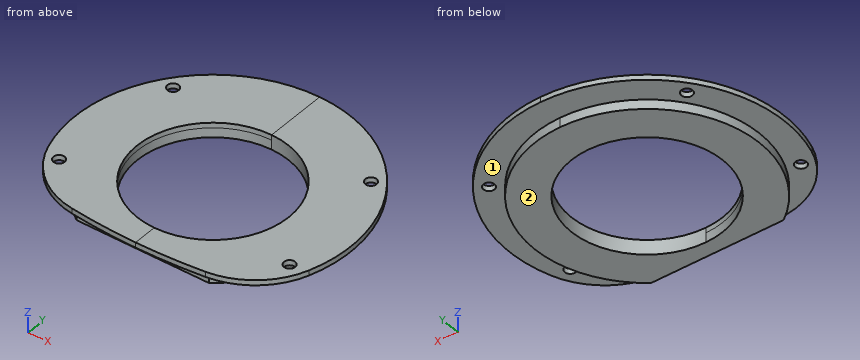
```python
from build123d import *

# Parameters (mm, degrees)
PAD_DEPTH    = 3
PAD001_DEPTH = 5.5
SKETCH002_R  = 3.25
POCKET_DEPTH = 5


with BuildPart() as part:
    # Sketch → Pad (new body)
    with BuildSketch(Plane.XY):
        with BuildLine():
            ThreePointArc((0, -44), (44, 0), (0, 44))
            Line((0, 80), (0, 44))
            ThreePointArc((75.734063, -25.775021), (65.046144, 46.572515), (0, 80))
            ThreePointArc((38.857167, -55.659898), (61.606206, -46.036578), (75.734063, -25.775021))
            ThreePointArc((0, -57.981235), (19.463222, -57.400384), (38.857167, -55.659898))
            Line((0, -57.981235), (0, -44))
        make_face()
    pad = extrude(amount=PAD_DEPTH)

    # Sketch001 (on Face7 of Pad) → Pad001 (join)
    with BuildSketch(Plane(origin=(0, 0, 0), x_dir=(1, 0, 0), z_dir=(0, 0, -1))):
        with BuildLine():
            ThreePointArc((0, -65.25), (62.028272, -20.249839), (38.5, 52.681235))
            Line((38.5, 52.681235), (0, 52.681235))
            Line((0, 44), (0, 52.681235))
            ThreePointArc((0, -44), (44, 0), (0, 44))
            Line((0, -44), (0, -65.25))
        make_face()
    pad001 = extrude(amount=PAD001_DEPTH)

    # Mirrored: Pad, Pad001 across Sketch V_Axis
    add(pad.mirror(Plane(origin=(0, 0, 0), x_dir=(0, 0, 1), z_dir=(1, 0, 0))))
    add(pad001.mirror(Plane(origin=(0, 0, 0), x_dir=(0, 0, 1), z_dir=(1, 0, 0))))

    # Sketch002 (on Face4 of Mirrored) → Pocket (cut)
    with BuildSketch(Plane(origin=(0, 0, 0), x_dir=(1, 0, 0), z_dir=(0, 0, -1))):
        with Locations((65.987317, 27.62811)):
            Circle(SKETCH002_R)
        with Locations((57.5, -44.318765)):
            Circle(SKETCH002_R)
        with Locations((-57.5, -44.318765)):
            Circle(SKETCH002_R)
        with Locations((-65.987317, 30.215763)):
            Circle(SKETCH002_R)
    extrude(amount=-POCKET_DEPTH, mode=Mode.SUBTRACT)


solid = part.part
```
Check sheet for the modelled part. Datum: model origin and axes. Units: mm. Face numbers are marked on the shaded views. A direction names the side the tool comes from. Round coordinates to 2 decimals unless told otherwise and drop trailing zeros. Order: outer loops, then holes, each group sorted by start corner. A loop starts at its lowest first (then second) coordinate and runs counter-clockwise, first axis right, second up. Notation, with made-up numbers: (-37.75, -31) - (-33.75, -31) arc R20 cw to (-33.75, -4) - close; hole circle Ø9 at (21, 54.25). An arc over 180 degrees is marked (long way). Write item = value, one per line.
Q1. Thickness scan on line 1 along X through (y, z) = (-25, 0.25); line 2 along X through (y, z) = (-5, -2.25); line 3 along Y through (x, z) = (-0.5, -4). Record the ranges inside material, lowest first.
Computed:
line_1 = -75.99 to -36.21, 36.21 to 64.08, 67.9 to 75.99
line_2 = -65.06 to -43.71, 43.71 to 65.06
line_3 = -52.68 to -44, 44 to 65.25
Q2. Tool access check on the marked faces 1 and 2. Record the directions out of +Z, -Z, +X, -X, +Y, -Y that give a thin tool (end or side, any length) a straight path to the whole face; none if there is none.
Computed:
face_1 = -Z
face_2 = -Z, +X, -X, +Y, -Y
Q3. Section check C-C (z = -3). Record the boundary of the cut face in (x, y).
Computed:
outline = (-38.5, -52.68) - (38.5, -52.68) arc R65.25 ccw (long way) to start; hole circle Ø88 at (0, 0)
Q4. Section check D-D (x = -67). Record the boundary of the cut face in (y, z), and give its area (3 significant figures).
Computed:
outline = (-40.86, 0) - (-33.3, 0) - (-33.3, 3) - (-40.86, 3) - close; (-27.13, 0) - (43.71, 0) - (43.71, 3) - (-27.13, 3) - close
area = 235 mm^2
Q5. Section check B-B (x = 42). Record the boundary of the cut face in (y, z), and give its area (3 significant figures).
Computed:
outline = (-55.17, 0) - (-49.94, 0) - (-49.94, -5.5) - (-13.11, -5.5) - (-13.11, 3) - (-55.17, 3) - close; (13.11, -5.5) - (49.94, -5.5) - (49.94, 0) - (68.09, 0) - (68.09, 3) - (13.11, 3) - close
area = 696 mm^2
Q6. Go/stop test with flat-tipped pins: pin 1 (4 mm diameter, centred on x = 18, z = 0, fed in from +Y); pin 2 (1.5 mm diameter, centred on y = 51.5, z = -4, fed in from -X); pin 3 (4 mm diameter, centred on y = 53.5, z = -0.5, fed in from +X); pin 4 (6 mm diameter, centred on x = 65.99, y = -27.63, fed in from +Z). Record where each tip stops, or that it passes through.
Computed:
pin_1 = 78.38
pin_2 = -41.01
pin_3 = 61.17
pin_4 = through
Q7. Section check A-A (y = 0). Record the boundary of the cut face in (x, z).
Computed:
outline = (-80, 0) - (-65.25, 0) - (-65.25, -5.5) - (-44, -5.5) - (-44, 3) - (-80, 3) - close; (44, -5.5) - (65.25, -5.5) - (65.25, 0) - (80, 0) - (80, 3) - (44, 3) - close
